from build123d import *

# Parameters (mm, degrees)
F0_W      = 13
F0_H      = 13
F1_DEPTH  = 5
F2_R      = 6
F3_DEPTH  = 25
F4_W      = 13
F4_H      = 1
F5_DEPTH  = 2
F6_W      = 1
F6_H      = 17
F7_DEPTH  = 2
F8_W      = 1
F8_H      = 15
F9_DEPTH  = 2
F10_DEPTH = 15
F11_DEPTH = 8
F12_DEPTH = 4
F13_W     = 10
F13_H     = 2
F14_DEPTH = 5


with BuildPart() as f1:
    # F0 (on Front) → F1 (new body)
    with BuildSketch(Plane.XZ):
        Rectangle(F0_W, F0_H)
    extrude(amount=F1_DEPTH)

    # F2 (on face) → F3 (cut)
    with BuildSketch(Plane(origin=(0, 0, 0), x_dir=(-1, 0, 0), z_dir=(0, 1, 0))):
        Circle(F2_R)
    extrude(amount=-F3_DEPTH, mode=Mode.SUBTRACT)

    # F4 (on face) → F5 (join)
    with BuildSketch(Plane.XY.offset(6.5)):
        with Locations((0, -4.5)):
            Rectangle(F4_W, F4_H)
    extrude(amount=F5_DEPTH)

    # F6 (on face) → F7 (join)
    with BuildSketch(Plane.YZ.offset(6.5)):
        with Locations((-4.5, 0)):
            Rectangle(F6_W, F6_H)
    extrude(amount=F7_DEPTH)

    # F8 (on face) → F9 (join)
    with BuildSketch(Plane(origin=(-6.5, 0, 0), x_dir=(0, -1, 0), z_dir=(-1, 0, 0))):
        with Locations((4.5, 1)):
            Rectangle(F8_W, F8_H)
    extrude(amount=F9_DEPTH)

    # F10 (add): a face of the model
    f10_faces = [f1.faces().sort_by_distance(p)[0] for p in [
        (6.5, -4.5, -7.5),
    ]]
    extrude(f10_faces, amount=F10_DEPTH)

    # F11 (add): a face of the model
    f11_faces = [f1.faces().sort_by_distance(p)[0] for p in [
        (0, -4, -8.2595836944),
    ]]
    extrude(f11_faces, amount=F11_DEPTH)

    # F12 (cut): a face of the model
    f12_faces = [f1.faces().sort_by_distance(p)[0] for p in [
        (6.3161522369, 0, 0),
    ]]
    extrude(f12_faces, amount=-F12_DEPTH, mode=Mode.SUBTRACT)

    # F13 (on face) → F14 (cut)
    with BuildSketch(Plane(origin=(0, 4, 0), x_dir=(-1, 0, 0), z_dir=(0, 1, 0))):
        with Locations((1.5, 7.5)):
            Rectangle(F13_W, F13_H)
    extrude(amount=-F14_DEPTH, mode=Mode.SUBTRACT)


solid = f1.part
Geometry: final body of the model. Coordinates: model frame, mm. A direction names the side the tool comes from. Round coordinates to 2 decimals unless told otherwise and drop trailing zeros. Write each loop counter-clockwise with the first axis right and the second up, starting at its lowest first coordinate (ties: lowest second). Pieces come first, ordered by that corner, then holes. Notation, with made-up numbers: M 18,21.5 L 76,21.5 A28 ccw 76,49.5 Z; hole C 35,27.5 d5. An arc over 180 degrees is marked long. Write item = value, one per line.
Item 1: Section query A-A on x = 0. Return loops of the section in (y, z).
Findings:
outline = M -5,-8.5 L 4,-8.5 L 4,-6.5 L -4,-6.5 L -4,-6 L -5,-6 Z; M -5,6 L -4,6 L -4,6.5 L -1,6.5 L -1,8.5 L -5,8.5 Z
Item 2: Section query C-C on y = -3.5. Return loops of the section in (x, z), then the cut area to 3 significant figures.
Findings:
outline = M -8.5,-8.5 L 8.5,-8.5 L 8.5,8.5 L -8.5,8.5 Z; hole M -6.5,-6.5 L 6.5,-6.5 L 6.5,6.5 L -6.5,6.5 Z
area = 120 mm^2
Item 3: Section query B-B on z = 0. Return loops of the section in (x, y), then the cut area to 3 significant figures.
Findings:
outline = M -8.5,-5 L -6,-5 L -6,-4 L -6.5,-4 L -6.5,4 L -8.5,4 Z; M 6,-5 L 8.5,-5 L 8.5,4 L 6.5,4 L 6.5,-4 L 6,-4 Z
area = 37.0 mm^2
Item 4: Pull-direction query (X, two-part tool) for faces 1 (the face through (1, -2, 6.5)), 2 (the face through (8.5, -1, 0)), 3 (the face through (0, -1, -8.5)); classes: pulls with the +X half, pulls with the -X half, needs draft (parallel to the pull), parting line crosses it, or undercut.
Findings:
face_1 = undercut
face_2 = pulls with the +X half
face_3 = needs draft
Item 5: Access query for faces 4 (the face through (3.5, 2, 7)), 5 (the face through (6.5, 0, 0)), 6 (the face through (-8.5, -1, 0)). Directions: +Z, -Z, +X, -X, +Y, -Y. A direction counts if a zero-diameter tool reaches every point of the face in a straight line with its end or side. Return the directions, or none.
Findings:
face_4 = +Z, +Y
face_5 = +Y
face_6 = +Z, -Z, -X, +Y, -Y
Item 6: Material intervals for line 1 along Z through (x, y) = (0, -4.6); line 2 along X through (y, z) = (3.5, 7.5); line 3 along X through (y, z) = (-1.5, -6), sorted ascending. Write a range as [from, to].
Findings:
line_1 = [-8.5, -6], [6, 8.5]
line_2 = [-8.5, -6.5], [3.5, 8.5]
line_3 = [-8.5, -6.5], [6.5, 8.5]
Item 7: Pin query (flat end, axial travel): P1, Ø2, axis at x = -1.5, z = 7, coming from the +Y side. Return the tip coordinate at first contact, or that it passes through.
Findings:
P1 = -1
Item 8: Section query D-D on y = -0.75. Return loops of the section in (x, z).
Findings:
outline = M -8.5,-8.5 L 8.5,-8.5 L 8.5,8.5 L 3.5,8.5 L 3.5,6.5 L 6.5,6.5 L 6.5,-6.5 L -6.5,-6.5 L -6.5,8.5 L -8.5,8.5 Z
